The listing builds one solid part. Answer for the finished solid, in the listing's coordinates (mm). A direction names the side the tool comes from. Give positions to 0.01 mm unless a question says otherwise; leave off trailing zeros. Order: outer loops, then holes, each group sorted by start corner. A loop starts at its lowest first (then second) coordinate and runs counter-clockwise, first axis right, second up. Notation, with made-up numbers: (12.5, 34) - (68.5, 34) arc R18 cw to (68.5, 69) - close; hole circle Ø4 at (-23, 57). An arc over 180 degrees is marked (long way). Use a Markdown table: item, result. Add a question column.
1) Find section A-A, the plane z = 72.5. Determine the outline of the cut face in (x, y).
2) Find section C-C, the plane y = -15.5. Determine the outline of the cut face in (x, z).
3) Find section B-B, the plane x = 28. Determine the outline of the cut face in (y, z).
4) Straight lines are drawn through the part: line 1 (Z direction, x = 67, y = -15.5); line 2 (X direction, y = -4.5, z = 69); line 3 (Z direction, x = 7.5, y = -19). For each, find the intervals that lie inside material, in ascending order.
5) Find section D-D, the plane x = 82. Determine the outline of the cut face in (y, z).
6) The mould has two halves that part along X. Classify faces 3 (the face through (5.436, -12.878, 70.963)), 4 (the face through (49, -25.4, 43)), 5 (the face through (100, -13, 42)), 6 (the face through (0, -13, 42)): released by +X, released by -X, zero draft, split by the parting line, or undercut.
7) For faces 1 (the face through (63.06, -17.501, 59.133)), 2 (the face through (49, -13, 85.391)), determine the directions among +Z, -Z, +X, -X, +Y, -Y from which every point of the face is accessible in a straight line to the end or side of a thin tool.
from build123d import *

# Parameters (mm, degrees)
F0_W     = 100
F0_H     = 85.3913038855
F1_DEPTH = 25.4
F2_R     = 13.1600821693
F3_DEPTH = 25.4
F4_R     = 8.3492682179
F5_DEPTH = 25.4
F6_DEPTH = 25.4
F7_DEPTH = 25.4


with BuildPart() as f1:
    # F0 (on Front) → F1 (new body)
    with BuildSketch(Plane.XZ):
        with Locations((50, 42.6956519428)):
            Rectangle(F0_W, F0_H)
    extrude(amount=F1_DEPTH)

    # F2 (on face) → F3 (cut)
    with BuildSketch(Plane.XZ.offset(25.4)):
        with Locations((18.5836926103, 70.3844353557)):
            Circle(F2_R)
    extrude(amount=-F3_DEPTH, mode=Mode.SUBTRACT)

    # F4 (on face) → F5 (cut)
    with BuildSketch(Plane.YZ.offset(100)):
        with Locations((-15.6908016652, 67.2837793827)):
            Circle(F4_R)
    extrude(amount=-F5_DEPTH, mode=Mode.SUBTRACT)

    # F6 (cut): a face of the model
    f6_faces = [f1.faces().sort_by_distance(p)[0] for p in [
        (74.6, -15.6908016652, 67.2837793827),
    ]]
    extrude(f6_faces, amount=-F6_DEPTH, mode=Mode.SUBTRACT)

    # F7 (cut): a face of the model
    f7_faces = [f1.faces().sort_by_distance(p)[0] for p in [
        (49.2, -15.6908016652, 67.2837793827),
    ]]
    extrude(f7_faces, amount=-F7_DEPTH, mode=Mode.SUBTRACT)


solid = f1.part
The answers:
| question | item | result |
|---|---|---|
| 1 | outline | (0, -25.4) - (5.59, -25.4) - (5.59, 0) - (0, 0) - close; (31.57, -25.4) - (100, -25.4) - (100, -22.21) - (31.57, -22.21) - close; (31.57, -9.17) - (100, -9.17) - (100, 0) - (31.57, 0) - close |
| 2 | outline | (0, 0) - (100, 0) - (100, 58.94) - (25.07, 58.94) arc R13.16 cw (long way) to (30.65, 75.63) - (100, 75.63) - (100, 85.39) - (0, 85.39) - close |
| 3 | outline | (-25.4, 0) - (0, 0) - (0, 61.19) - (-9.98, 61.19) arc R8.35 cw to (-21.4, 61.19) - (-25.4, 61.19) - close; (-25.4, 79.58) - (0, 79.58) - (0, 85.39) - (-25.4, 85.39) - close |
| 4 | line 1 | 0 to 58.94, 75.63 to 85.39 |
| 4 | line 2 | 0 to 5.5, 31.67 to 100 |
| 4 | line 3 | 0 to 63.29, 77.48 to 85.39 |
| 5 | outline | (-25.4, 0) - (0, 0) - (0, 85.39) - (-25.4, 85.39) - close; hole circle Ø16.7 at (-15.69, 67.28) |
| 6 | face 3 | undercut |
| 6 | face 4 | zero draft |
| 6 | face 5 | released by +X |
| 6 | face 6 | released by -X |
| 7 | face 1 | +X |
| 7 | face 2 | +Z, +X, -X, +Y, -Y |
